The drawing under review shows one solid part. Ordinate dimensions are in mm from its lowest x, y, z. A direction names the side the tool comes from. Round coordinates to 2 decimals unless told otherwise and drop trailing zeros. Order: outer loops, then holes, each group sorted by start corner. A loop starts at its lowest first (then second) coordinate and runs counter-clockwise, first axis right, second up. Notation, with made-up numbers: M -32,34 L 24,34 A23 ccw 24,73 Z; hole C -37.75,-10 d1. An arc over 180 degrees is marked long. Answer as a JSON object with one key per item and string values. Group by question number.
1) To check wall thickness, follow line 1 (Z direction, x = 27.9, y = 13.5); line 2 (X direction, y = 13.25, z = 27.5). State the ranges of each line that lie inside material, in increasing order.
2) Consider section C-C, the plane z = 26.25. Write out the cut boundary in (x, y), then the cut area to 3 significant figures.
3) Consider section B-B, the plane z = 15. Write out the cut boundary in (x, y), then the cut area to 3 significant figures.
4) Consider section A-A, the plane y = 13.5. Write out the cut boundary in (x, z).
5) For the marked faces 1 and 2, list the 3-axis set-ups (+Z, -Z, +X, -X, +Y, -Y) from which the entire face can be reached by the end or side of a thin tool; tool diameter is ignored.
6) Insertion check: pin 1 Ø8 at (y, z) = (13, 4) entering from -X. The pin has a flat end and moves straight along its axis. Give the tip position at first contact, or say it passes through.
7) Consider section D-D, the plane x = 15.25. Write out the cut boundary in (y, z), then the cut area to 3 significant figures.
8) The part is to be moulded in two halves that separate along Y. For the marked faces 3, 4 and 5, say which applies: +Y half, -Y half, draft (parallel to the pull), parting line (faces both ways), or undercut.
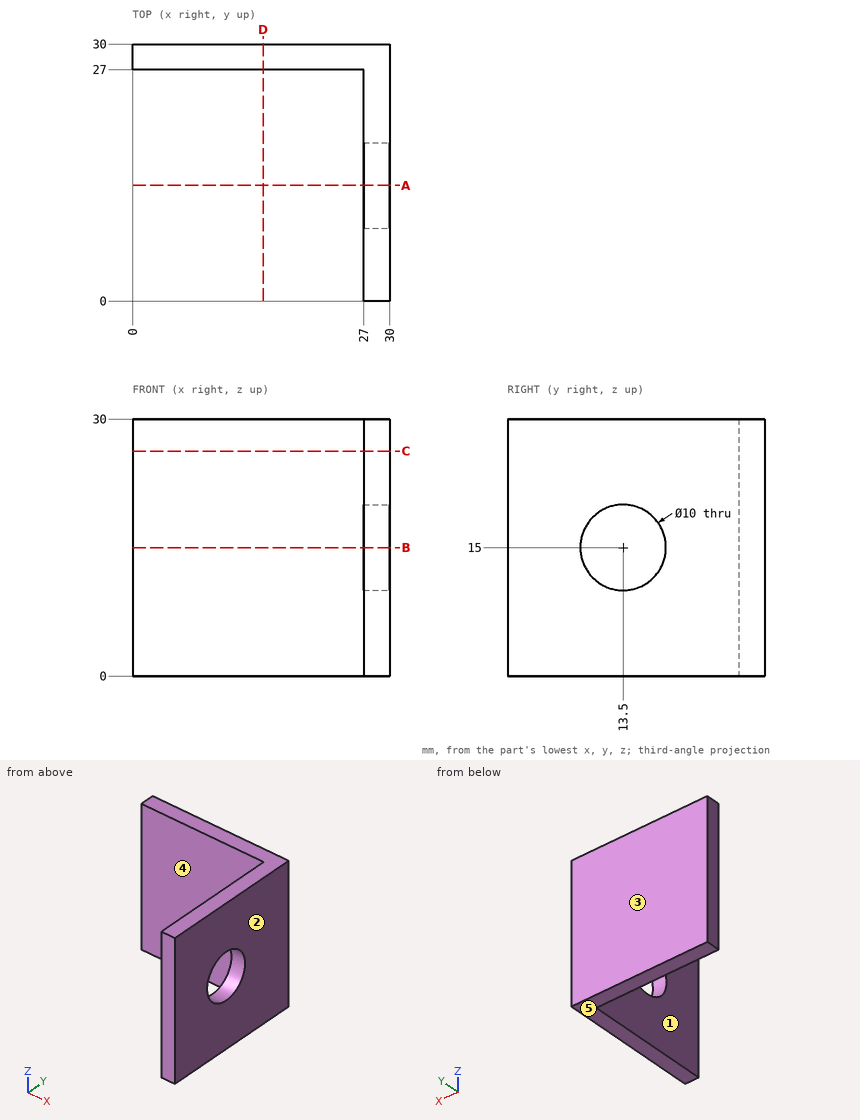
Results list:
{
 "1": {"line 1": "0 to 10, 20 to 30", "line 2": "27 to 30"},
 "2": {"outline": "M 0,27 L 27,27 L 27,0 L 30,0 L 30,30 L 0,30 Z", "area": "171 mm^2"},
 "3": {"outline": "M 0,27 L 27,27 L 27,18.5 L 30,18.5 L 30,30 L 0,30 Z; M 27,0 L 30,0 L 30,8.5 L 27,8.5 Z", "area": "141 mm^2"},
 "4": {"outline": "M 27,0 L 30,0 L 30,10 L 27,10 Z; M 27,20 L 30,20 L 30,30 L 27,30 Z"},
 "5": {"face 1": "+Z, -Z, -X, -Y", "face 2": "+Z, -Z, +X, +Y, -Y"},
 "6": {"pin 1": "x = 27"},
 "7": {"outline": "M 27,0 L 30,0 L 30,30 L 27,30 Z", "area": "90.0 mm^2"},
 "8": {"face 3": "+Y half", "face 4": "-Y half", "face 5": "draft"}
}
